Work out the finished part from the listing and answer in its coordinate system (mm). Face numbers are marked on the shaded views. A direction names the side the tool comes from. Round coordinates to 2 decimals unless told otherwise and drop trailing zeros. Order: outer loops, then holes, each group sorted by start corner. A loop starts at its lowest first (then second) coordinate and runs counter-clockwise, first axis right, second up. Notation, with made-up numbers: M 1,10.25 L 36,10.25 A29 cw 36,30.25 Z; hole C -34.5,-18 d6. An arc over 180 degrees is marked long. Answer as a JSON object with one key per item and string values. Group by question number.
from build123d import *

# Parameters (mm, degrees)
SKETCH1_R            = 1
BASE_EXTRUDE_DEPTH   = 1
BOSS_EXTRUDE7_DEPTH  = 1
CIRPATTERN1_COUNT    = 2
BOSS_EXTRUDE8_DEPTH  = 1
SKETCH10_R           = 3
BOSS_EXTRUDE9_DEPTH  = 4
CHAMFER1_SIZE        = 1
CUT_EXTRUDE1_DEPTH   = 0.5
SKETCH14_R           = 2.5
BOSS_EXTRUDE10_DEPTH = 0.5


with BuildPart() as part:
    # Sketch1 → Base Extrude (new body)
    with BuildSketch(Plane(origin=(0, 0, 0), x_dir=(1, 0, 0), z_dir=(0, 1, 0))):
        with BuildLine():
            Line((0, 8), (16, 8))
            ThreePointArc((16, 8), (22.821901857, 4.178714521), (23.126695088, -3.634586238))
            ThreePointArc((23.126695088, -3.634586238), (23.424621202, -7.424621202), (19.634586238, -7.126695088))
            ThreePointArc((19.634586238, -7.126695088), (17.86901569, -7.778610438), (16, -8))
            Line((16, -8), (0, -8))
            ThreePointArc((0, -8), (-6.821901857, -4.178714521), (-7.126695088, 3.634586238))
            ThreePointArc((-7.126695088, 3.634586238), (-7.424621202, 7.424621202), (-3.634586238, 7.126695088))
            ThreePointArc((-3.634586238, 7.126695088), (-1.86901569, 7.778610438), (0, 8))
        make_face()
        with Locations(Location((-5.656854249, 5.656854249, 0), (0, 0, 270))):
            Circle(SKETCH1_R, mode=Mode.SUBTRACT)
        with Locations(Location((21.656854249, -5.656854249, 0), (0, 0, 270))):
            Circle(SKETCH1_R, mode=Mode.SUBTRACT)
    extrude(amount=BASE_EXTRUDE_DEPTH)

    # Sketch4 → Boss-Extrude7 (add)
    with BuildSketch(Plane(origin=(0, 1, 0), x_dir=(1, 0, 0), z_dir=(0, 1, 0))):
        with BuildLine():
            Line((-4.292206887, 5.529643754), (-4.866905142, 6.270026662))
            ThreePointArc((-4.866905142, 6.270026662), (-6.37503243, 6.352713503), (-6.244790585, 4.847947045))
            ThreePointArc((-6.244790585, 4.847947045), (-6.079062433, 3.80031439), (-7.126695088, 3.634586238))
            ThreePointArc((-7.126695088, 3.634586238), (-7.424621202, 7.424621202), (-3.634586238, 7.126695088))
            ThreePointArc((-3.634586238, 7.126695088), (-1.86901569, 7.778610438), (0, 8))
            ThreePointArc((0, 8), (5.656854249, 5.656854249), (8, 0))
            ThreePointArc((8, 0), (8.005634917, -0.300211458), (8.02253173, -0.6))
            Line((8.02253173, -0.6), (6.97423831, -0.6))
            ThreePointArc((6.97423831, -0.6), (3.3453634, 6.148865239), (-4.292206887, 5.529643754))
        make_face()
        with BuildLine():
            ThreePointArc((-7, 0), (-2.291287847, -6.614378278), (5.5, -4.330127019))
            ThreePointArc((5.5, -4.330127019), (6.20215193, -4.246564663), (6.285714286, -4.948716593))
            ThreePointArc((6.285714286, -4.948716593), (3.493584639, -7.196865038), (0, -8))
            ThreePointArc((0, -8), (-5.656854249, -5.656854249), (-8, 0))
            ThreePointArc((-8, 0), (-7.5, 0.5), (-7, 0))
        make_face()
    boss_extrude7 = extrude(amount=BOSS_EXTRUDE7_DEPTH)

    # CirPattern1: Boss-Extrude7 ×2 about axis
    cirpattern1_axis = Axis((8, 0, 0), (0, 1, 0))
    for i in range(1, CIRPATTERN1_COUNT):
        add(boss_extrude7.rotate(cirpattern1_axis, i * 360 / CIRPATTERN1_COUNT))

    # Sketch9 → Boss-Extrude8 (add)
    with BuildSketch(Plane(origin=(0, 1, 0), x_dir=(1, 0, 0), z_dir=(0, 1, 0))):
        with BuildLine():
            Line((12.127016654, 7), (3.872983346, 7))
            ThreePointArc((3.872983346, 7), (2, 7.745966692), (0, 8))
            Line((0, 8), (16, 8))
            ThreePointArc((16, 8), (14, 7.745966692), (12.127016654, 7))
        make_face()
        with BuildLine():
            Line((3.872983346, -7), (12.127016654, -7))
            ThreePointArc((12.127016654, -7), (14, -7.745966692), (16, -8))
            Line((16, -8), (0, -8))
            ThreePointArc((0, -8), (2, -7.745966692), (3.872983346, -7))
        make_face()
    extrude(amount=BOSS_EXTRUDE8_DEPTH)

    # Sketch10 → Boss-Extrude9 (add)
    with BuildSketch(Plane(origin=(0, 1, 0), x_dir=(1, 0, 0), z_dir=(0, 1, 0))):
        with Locations(Location((16, 0, 0), (0, 0, 270))):
            Circle(SKETCH10_R)
        with Locations(Location((0, 0, 0), (0, 0, 270))):
            Circle(SKETCH10_R)
    extrude(amount=BOSS_EXTRUDE9_DEPTH)

    # Chamfer1
    chamfer1_edges = [part.edges().sort_by_distance(p)[0] for p in [
        (16, 1, -3),
        (0, 1, -3),
    ]]
    chamfer(chamfer1_edges, length=CHAMFER1_SIZE)

    # Sketch12 → Back Cavity (revolve, cut)
    with BuildSketch(Plane.XY, mode=Mode.PRIVATE) as back_cavity_sk:
        Polygon((0, 1.75), (2.5, 1.75), (3.5, 0.5), (3.5, 0), (0, 0), align=None)
    back_cavity = revolve(back_cavity_sk.sketch.rotate(Axis((0, 3.203039839, 0), (0, -1, 0)), 90), axis=Axis((0, 3.203039839, 0), (0, -1, 0)), mode=Mode.SUBTRACT)

    # Mirror1: Back Cavity across plane
    add(back_cavity.mirror(Plane(origin=(8, 0, 0), x_dir=(0, 0, 1), z_dir=(1, 0, 0))), mode=Mode.SUBTRACT)

    # Sketch13 → Cut-Extrude1 (cut)
    with BuildSketch(Plane.XZ):
        with BuildLine():
            Line((3.354101966, 1), (12.645898034, 1))
            ThreePointArc((12.645898034, 1), (12.5, 0), (12.645898034, -1))
            Line((12.645898034, -1), (3.354101966, -1))
            ThreePointArc((3.354101966, -1), (3.5, 0), (3.354101966, 1))
        make_face()
        with BuildLine():
            Line((-1, 3.354101966), (-1, 7.937253933))
            ThreePointArc((-1, 7.937253933), (-0.5009833, 7.984298074), (0, 8))
            Line((0, 8), (1, 8))
            Line((1, 8), (1, 3.354101966))
            ThreePointArc((1, 3.354101966), (0, 3.5), (-1, 3.354101966))
        make_face()
        with BuildLine():
            Line((16, -8), (15, -8))
            Line((15, -8), (15, -3.354101966))
            ThreePointArc((15, -3.354101966), (16, -3.5), (17, -3.354101966))
            Line((17, -3.354101966), (17, -7.937253933))
            ThreePointArc((17, -7.937253933), (16.5009833, -7.984298074), (16, -8))
        make_face()
        with BuildLine():
            Line((-1, -3.354101966), (-1, -7.937253933))
            ThreePointArc((-1, -7.937253933), (-0.5009833, -7.984298074), (0, -8))
            Line((0, -8), (1, -8))
            Line((1, -8), (1, -3.354101966))
            ThreePointArc((1, -3.354101966), (0, -3.5), (-1, -3.354101966))
        make_face()
        with BuildLine():
            Line((15, 3.354101966), (15, 8))
            Line((15, 8), (16, 8))
            ThreePointArc((16, 8), (16.5009833, 7.984298074), (17, 7.937253933))
            Line((17, 7.937253933), (17, 3.354101966))
            ThreePointArc((17, 3.354101966), (16, 3.5), (15, 3.354101966))
        make_face()
    extrude(amount=-CUT_EXTRUDE1_DEPTH, mode=Mode.SUBTRACT)

    # Sketch14 → Boss-Extrude10 (add)
    with BuildSketch(Plane.XZ.offset(-1.75)):
        with Locations(Location((0, 0, 0), (0, 0, 270))):
            Circle(SKETCH14_R)
    boss_extrude10 = extrude(amount=BOSS_EXTRUDE10_DEPTH)

    # Mirror2: Boss-Extrude10 across plane
    add(boss_extrude10.mirror(Plane(origin=(8, 0, 0), x_dir=(0, 0, 1), z_dir=(1, 0, 0))))


solid = part.part
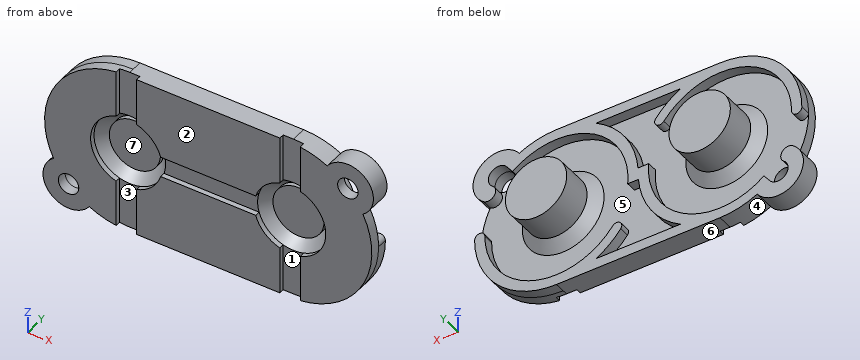
Item 1: Find section B-B (x = -7.5). Give the vertices of the cut face in (y, z), and give its area (3 significant figures).
Item 2: The mould has two halves that part along X. Classify the marked faces 1 and 2: +X half, -X half, draft (parallel to the pull), parting line (faces both ways), or undercut.
Item 3: Each of these flat-tipped pins is pushed along its axis until it touches: pin 1 (1 mm diameter, centred on y = 1, z = 2, fed in from -X); pin 2 (1.6 mm diameter, centred on x = -5.66, z = -5.66, fed in from -Y); pin 3 (3 mm diameter, centred on x = 19.5, y = 2, fed in from -Z); pin 4 (5.5 mm diameter, centred on x = 16.5, z = 0.5, fed in from -Y). Where does it stop, or does it pass through?
Item 4: Consider L1, parallel to Z at x = 9, y = 0.35; L2, parallel to X at y = 4.35, z = 0; L3, parallel to Y at x = 20, z = -2.25. Determine where each line is inside the solid, lowest interval first.
Item 5: A tool of negligible diameter and unlimited length cuts with its end or side. For the marked faces 3, 4, 5, 6 and 7, from which of +Z, -Z, +X, -X, +Y, -Y can it reach the whole face along a straight path? Write none if from no direction.
Item 6: Find section A-A (y = 2.85). Give the vertices of the cut face in (x, z).
Responses:
{
 "1": {"outline": "M 0,-7.35 L 2,-7.35 L 2,-3.97 L 0,-3.97 Z; M 0,-2.78 L 1,-2.78 L 1,-0.5 L 2,-0.5 L 2,2.78 L 0,2.78 Z", "area": "15.6 mm^2"},
 "2": {"face 1": "undercut", "face 2": "draft"},
 "3": {"pin 1": "stops at x = -7.86", "pin 2": "passes through", "pin 3": "stops at z = -7.75", "pin 4": "stops at y = 0.55"},
 "4": {"L1": "z = -8 to -1, 1 to 8", "L2": "x = -3 to 3, 13 to 19", "L3": "y = 0 to 1"},
 "5": {"face 3": "+Z, -Z, -Y", "face 4": "-Z, +Y, -Y", "face 5": "+Y", "face 6": "-Z, +X, +Y, -Y", "face 7": "-Y"},
 "6": {"outline": "C 0,0 d6; C 16,0 d6"}
}
